Check sheet for the modelled part. Datum: model origin and axes. Units: mm. A direction names the side the tool comes from. Round coordinates to 2 decimals unless told otherwise and drop trailing zeros. Loops run counter-clockwise (first coordinate to the right, second up) from the corner with the lowest first, then second, coordinate; pieces in that order, holes last. Notation, with made-up numbers: M 63,25.5 L 77,25.5 A23 ccw 77,62.5 Z; hole C 10.5,46.25 d2. An arc over 180 degrees is marked long. One line per question, with ' | ' between items. Start each with the question number.
(1) Thickness scan on probe 1 along Y at (x, z) = (71, -8); probe 2 along X at (y, z) = (1.3, -6.35) (3 decimals); probe 3 along X at (y, z) = (1.25, -6.35) (1 decimal). Record the ranges inside material, lowest first. Write a range as [from, to].
(2) Section check A-A (x = 6.35). Record the boundary of the cut face in (y, z) (3 decimals), and give its area (3 significant figures).
(3) Section check D-D (x = 69.5). Record the boundary of the cut face in (y, z).
(4) Draft check along X on faces 4 (the face through (63.447, 56.001, -6.439)), 5 (the face through (4.84, 1.93, -5.19)), 6 (the face through (71.46, 54.27, -5.62)), 7 (the face through (4, 0, -6)). Enter one of: +X half, -X half, draft (parallel to the pull), parting line (faces both ways), or undercut.
(5) Tool access check on faces 1 (the face through (4, 3.81, -6)), 2 (the face through (76.048, 54, -6)), 3 (the face through (71, 52.388, -8)). Record the directions out of +Z, -Z, +X, -X, +Y, -Y that give a thin tool (end or side, any length) a straight path to the whole face; none if there is none.
(6) Section check B-B (z = -6.35). Count the separate pieces of the cut face and the enclosed holes in it, and give its area (3 significant figures).
(7) Section check C-C (z = -1.5). Record the boundary of the cut face in (x, y).
(8) Go/stop test with flat-tipped pins: P1, Ø6, axis at x = 8, z = -7.5, coming from the +Y side; P2, Ø3, axis at x = 61.5, z = -2, coming from the +Y side; P3, Ø4, axis at y = 25, z = -7, coming from the -X side. Record where each tip stops, or that it passes through.
```python
from build123d import *

# Parameters (mm, degrees)
SKETCH1_W               = 12.7
SKETCH1_H               = 12.7
BOSS_EXTRUDE1_DEPTH     = 3.81
BOSS_EXTRUDE2_DEPTH     = 12.7
FILLET1_R               = 2.54
SKETCH6_R               = 1.905
CUT_EXTRUDE1_DEPTH      = 53.3875
CUT_EXTRUDE1_DEPTH_BACK = 4.81


with BuildPart() as part:
    # Sketch1 → Boss-Extrude1 (new body)
    with BuildSketch(Plane(origin=(0, 0, 0), x_dir=(1, 0, 0), z_dir=(0, 1, 0))):
        with Locations((6.35, 6.35)):
            Rectangle(SKETCH1_W, SKETCH1_H)
    extrude(amount=BOSS_EXTRUDE1_DEPTH)

    # Sketch2 → Boss-Extrude2 (add)
    with BuildSketch(Plane.XY):
        Polygon((12.7, 0), (63.348255925, 52.3875), (76.048255925, 52.3875), (76.048255925, 56.1975), (63.348255925, 56.1975), (12.7, 3.81), align=None)
    extrude(amount=-BOSS_EXTRUDE2_DEPTH)

    # Fillet1
    fillet1_edges = [part.edges().sort_by_distance(p)[0] for p in [
        (12.7, 3.81, -6.35),
        (63.348255925, 56.1975, -6.35),
        (63.348255925, 52.3875, -6.35),
        (12.7, 0, -6.35),
    ]]
    fillet(fillet1_edges, radius=FILLET1_R)

    # Sketch6 → Cut-Extrude1 (cut, two sides)
    with BuildSketch(Plane(origin=(0, 3.81, 0), x_dir=(1, 0, 0), z_dir=(0, 1, 0))) as cut_extrude1_sk:
        with Locations((6.35, 6.35)):
            Circle(SKETCH6_R)
        with Locations((69.698255925, 6.35)):
            Circle(SKETCH6_R)
    extrude(amount=CUT_EXTRUDE1_DEPTH, mode=Mode.SUBTRACT)
    extrude(cut_extrude1_sk.sketch, amount=-CUT_EXTRUDE1_DEPTH_BACK, mode=Mode.SUBTRACT)


solid = part.part
```
The answers:
1) probe 1: [52.39, 56.2] | probe 2: [0, 4.445], [8.255, 13.957] | probe 3: [0, 4.4], [8.3, 13.9]
2) outline: M 0,-12.7 L 3.81,-12.7 L 3.81,-8.255 L 0,-8.255 Z; M 0,-4.445 L 3.81,-4.445 L 3.81,0 L 0,0 Z | area: 33.9 mm²
3) outline: M 52.39,-12.7 L 56.2,-12.7 L 56.2,-8.24 L 52.39,-8.24 Z; M 52.39,-4.46 L 56.2,-4.46 L 56.2,0 L 52.39,0 Z
4) face 4: -X half | face 5: undercut | face 6: undercut | face 7: draft
5) face 1: +Z, -Z, -X, +Y | face 2: +Z, -Z, +X, +Y, -Y | face 3: +Z, -Z, +X, -Y
6) separate pieces: 3 | enclosed holes: 0 | area: 261 mm²
7) outline: M 0,0 L 11.62,0 A2.54 ccw 13.45,0.77 L 62.6,51.61 A2.54 cw 64.43,52.39 L 76.05,52.39 L 76.05,56.2 L 64.43,56.2 A2.54 ccw 62.6,55.42 L 13.45,4.58 A2.54 cw 11.62,3.81 L 0,3.81 Z
8) P1: y = 3.81 | P2: y = 55.76 | P3: x = 31.25
